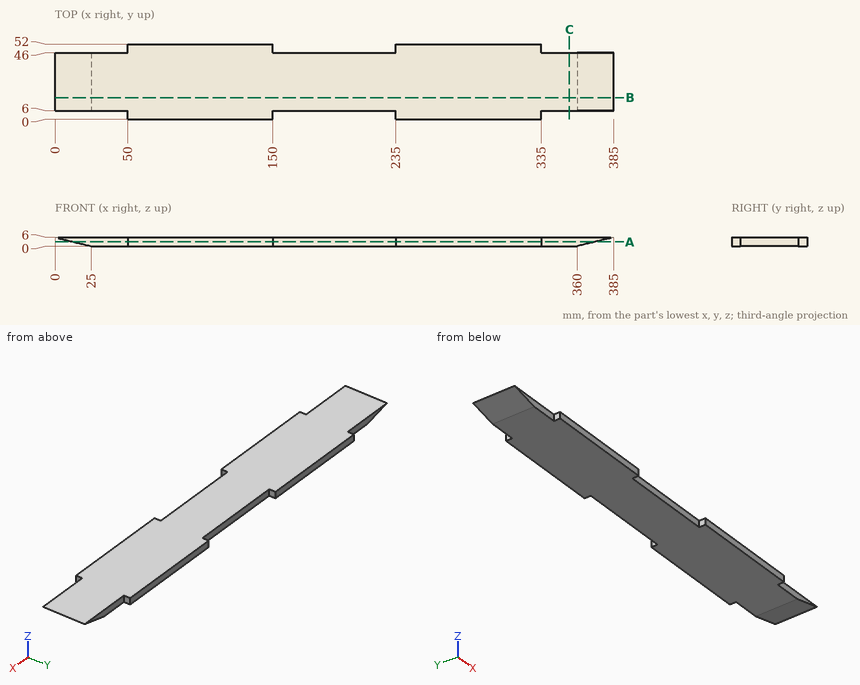
Verification items for this drawing (mm, ordinates from the low corner). Round coordinates to 2 decimals unless told otherwise and drop trailing zeros. Order: outer loops, then holes, each group sorted by start corner. A loop starts at its lowest first (then second) coordinate and runs counter-clockwise, first axis right, second up.
1) Cross-section at B-B, the plane y = 15. Record the cut outline in (x, z), plus the area to 3 significant figures.
Geometry says:
outline: (0, 6) - (25, 0) - (360, 0) - (385, 6) - close
area: 2,160 mm2
2) Depth check by flat-ended pin: pin 1 (1.8 mm diameter, centred on y = 49, z = 2, fed in from +X); pin 2 (3 mm diameter, centred on x = 177, z = 1, fed in from -Y); pin 3 (1.8 mm diameter, centred on x = 367.5, z = 4, fed in from +Y). Enter the tip coordinate at first touch or a pass-through.
Geometry says:
pin 1: stops at x = 335
pin 2: stops at y = 6
pin 3: stops at y = 46
3) Material ranges on line 1 (X direction, y = 4, z = 4.4); line 2 (Y direction, x = 25, z = 0.55), recorded low to high.
Geometry says:
line 1: x = 50 to 150, 235 to 335
line 2: y = 6 to 46
4) Cross-section at C-C, the plane x = 354.5. Record the cut outline in (y, z).
Geometry says:
outline: (6, 0) - (46, 0) - (46, 6) - (6, 6) - close
5) Cross-section at A-A, the plane z = 3. Record the cut outline in (x, y), plus the area to 3 significant figures.
Geometry says:
outline: (12.5, 6) - (50, 6) - (50, 0) - (150, 0) - (150, 6) - (235, 6) - (235, 0) - (335, 0) - (335, 6) - (372.5, 6) - (372.5, 46) - (335, 46) - (335, 52) - (235, 52) - (235, 46) - (150, 46) - (150, 52) - (50, 52) - (50, 46) - (12.5, 46) - close
area: 16,800 mm2
